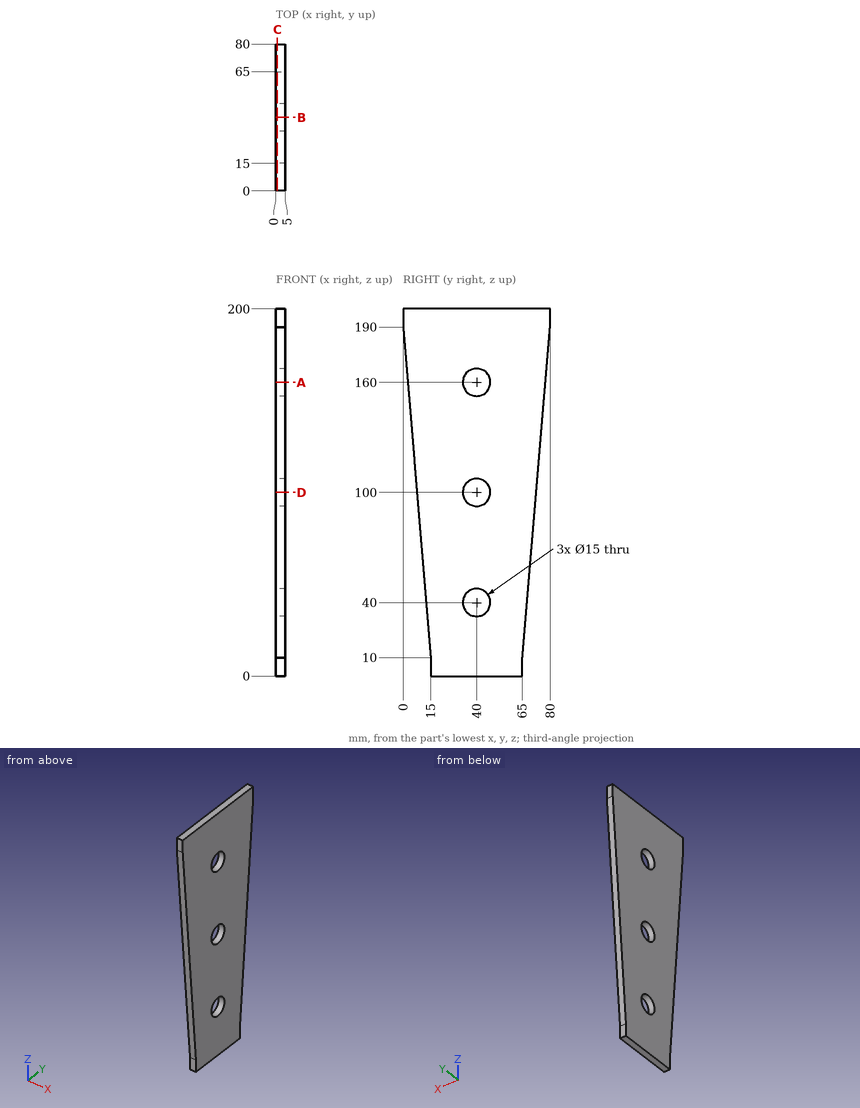
Part print with two shaded views. Sizes in mm from the minimum x, y, z corner. Coordinates: 2 decimals unless noted, no trailing zeros. Write each loop counter-clockwise with the first axis right and the second up, starting at its lowest first coordinate (ties: lowest second). Pieces come first, ordered by that corner, then holes. Notation, with made-up numbers: (33.25, 62.5) -> (80.25, 62.5) arc R32 cw to (80.25, 91.5) -> close; hole circle Ø10 at (79, 71). An arc over 180 degrees is marked (long way). Return JSON: item names as keys, results as strings. Group by question number.
Q1. Cut at B-B, the plane y = 40. Give the cut face in (x, z).
Q2. Drill centre lines: line 1 (Z direction, x = 4.4, y = 41.5); line 2 (Y direction, x = 3.45, z = 100); line 3 (Y direction, x = 2.85, z = 36.5). Where is each one in solid material? Low to high.
Q3. Cut at A-A, the plane z = 160. Give the cut face in (x, y).
Q4. Cut at C-C, the plane x = 0.75. Give the cut face in (y, z), then the cut area to 3 significant figures.
Q5. Flat gauge pins, fed straight in: pin 1 (2.5 mm diameter, centred on x = 3.5, z = 7, fed in from +Y); pin 2 (1.5 mm diameter, centred on x = 1, z = 92.5, fed in from -Y); pin 3 (1.5 mm diameter, centred on x = 2, z = 3.5, fed in from -Y). Where does each tip first touch, or does it go through?
Q6. Cut at D-D, the plane z = 100. Give the cut face in (x, y).
Returned:
{
 "1": {"outline": "(0, 0) -> (5, 0) -> (5, 32.5) -> (0, 32.5) -> close; (0, 47.5) -> (5, 47.5) -> (5, 92.5) -> (0, 92.5) -> close; (0, 107.5) -> (5, 107.5) -> (5, 152.5) -> (0, 152.5) -> close; (0, 167.5) -> (5, 167.5) -> (5, 200) -> (0, 200) -> close"},
 "2": {"line 1": "z = 0 to 32.65, 47.35 to 92.65, 107.35 to 152.65, 167.35 to 200", "line 2": "y = 7.5 to 32.5, 47.5 to 72.5", "line 3": "y = 12.79 to 33.37, 46.63 to 67.21"},
 "3": {"outline": "(0, 2.5) -> (5, 2.5) -> (5, 32.5) -> (0, 32.5) -> close; (0, 47.5) -> (5, 47.5) -> (5, 77.5) -> (0, 77.5) -> close"},
 "4": {"outline": "(0, 190) -> (15, 10) -> (15, 0) -> (65, 0) -> (65, 10) -> (80, 190) -> (80, 200) -> (0, 200) -> close; hole circle Ø15 at (40, 40); hole circle Ø15 at (40, 100); hole circle Ø15 at (40, 160)", "area": "12,500 mm2"},
 "5": {"pin 1": "stops at y = 65", "pin 2": "stops at y = 8.06", "pin 3": "stops at y = 15"},
 "6": {"outline": "(0, 7.5) -> (5, 7.5) -> (5, 32.5) -> (0, 32.5) -> close; (0, 47.5) -> (5, 47.5) -> (5, 72.5) -> (0, 72.5) -> close"}
}
